Work out the finished part from the listing and answer in its coordinate system (mm). Face numbers are marked on the shaded views. Give positions to 0.01 mm unless a question says otherwise; leave off trailing zeros. Order: outer loops, then holes, each group sorted by start corner. A loop starts at its lowest first (then second) coordinate and runs counter-clockwise, first axis right, second up. Notation, with made-up numbers: (48, -4) -> (86, -4) arc R35 ccw to (86, 34) -> close; hole circle Ø8 at (21.25, 64). An arc over 180 degrees is marked (long way). Answer as CSV lines item,"result". Start each with the question number.
1. A cutting plane is placed at A-A (z = 17). Give the vertices of the cut face in (x, y).
2. Find the intervals of material crossed by L1, parallel to Z at x = -4, y = 11.5; L2, parallel to Z at x = 10.5, y = -4; L3, parallel to Z at x = -5, y = 4.5, in increasing order.
3. For a pull along Z with two mould halves and no side action, classify the marked faces 1, 2, 3 and 4 as released by +Z, released by -Z, zero draft, split by the parting line, or undercut.
4. Flat-ended cylindrical pins translate along their axes: pin 1 (3 mm diameter, centred on x = -3.5, y = -5.5, fed in from +Z); pin 2 (6 mm diameter, centred on y = -3, z = 51, fed in from +X); pin 3 (10 mm diameter, centred on y = 1.5, z = 49.5, fed in from +X). Find the tip coordinate at first contact, or state that the pin passes through.
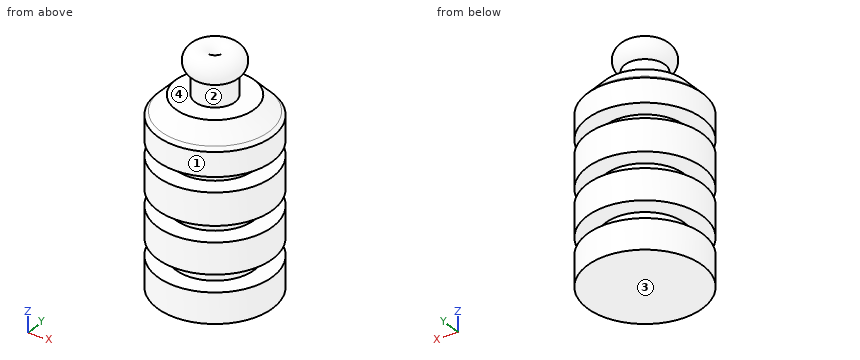
from build123d import *


with BuildPart() as f1:
    # F0 (on Front) → F1 (revolve)
    with BuildSketch(Plane.XZ):
        Polygon((0, 54.25334), (0, 0), (15.178914, 0), (15.178914, 7.965172), (10.369752, 7.965172), (10.369752, 12.47376), (15.178914, 12.47376), (15.178914, 20.589218), (10.369752, 20.589218), (10.369752, 24.797235), (15.178914, 24.797235), (15.178914, 33.213265), (10.369752, 33.213265), (10.369752, 37.120707), (15.178914, 37.120707), (15.178914, 43.432731), (14.304863, 44.36141), (10.369752, 48.542466), (5.26002, 48.542466), (5.26002, 54.25334), (2.63001, 54.25334), align=None)
        with BuildLine():
            ThreePointArc((5.26002, 54.25334), (3.945015, 60.362486), (2.63001, 54.25334))
            Line((2.63001, 54.25334), (5.26002, 54.25334))
        make_face()
    revolve(axis=Axis((0, 0, 27.12667), (0, 0, -1)))


solid = f1.part
Answer sheet:
1,outline,"circle Ø30.36 at (0, 0)"
2,L1,"z = 0 to 7.97, 12.47 to 20.59, 24.8 to 33.21, 37.12 to 46.62"
2,L2,"z = 0 to 7.97, 12.47 to 20.59, 24.8 to 33.21, 37.12 to 47.62"
2,L3,"z = 0 to 48.54, 55.59 to 58.74"
3,face 1,"zero draft"
3,face 2,"undercut"
3,face 3,"released by -Z"
3,face 4,"undercut"
4,pin 1,"stops at z = 60.18"
4,pin 2,"stops at x = 10.55"
4,pin 3,"stops at x = 14.12"
